```python
from build123d import *

# Parameters (mm, degrees)
SZKIC1_W                                            = 110
SZKIC1_H                                            = 80
DODANIE_WYCI_GNI_CIE1_DEPTH                         = 20
SZKIC4_W                                            = 20
SZKIC4_H                                            = 140
DODANIE_WYCI_GNI_CIE2_DEPTH                         = 75
WYTNIJ_WYCI_GNI_CIE2_DEPTH                          = 56
WYTNIJ_WYCI_GNI_CIE2_DEPTH_BACK                     = 56
POG_BIENIE_WALCOWE_POD_M5_WKR_T_Z_BEM_W_D           = 5.8
POG_BIENIE_WALCOWE_POD_M5_WKR_T_Z_BEM_W_CBORE_D     = 10
POG_BIENIE_WALCOWE_POD_M5_WKR_T_Z_BEM_W_CBORE_DEPTH = 5.4
WYTNIJ_WYCI_GNI_CIE3_DEPTH                          = 111
SZKIC19_R                                           = 2.65
WYTNIJ_WYCI_GNI_CIE4_DEPTH                          = 20
WYTNIJ_WYCI_GNI_CIE5_DEPTH                          = 5
WYTNIJ_WYCI_GNI_CIE6_DEPTH                          = 10


with BuildPart() as part:
    # Szkic1 → Dodanie-wyciągnięcie1 (new body)
    with BuildSketch(Plane.XY):
        Rectangle(SZKIC1_W, SZKIC1_H)
    extrude(amount=DODANIE_WYCI_GNI_CIE1_DEPTH)

    # Szkic4 → Dodanie-wyciągnięcie2 (add)
    with BuildSketch(Plane.XY.offset(20)):
        with Locations((-45, 0)):
            Rectangle(SZKIC4_W, SZKIC4_H)
        with Locations((45, 0)):
            Rectangle(SZKIC4_W, SZKIC4_H)
    extrude(amount=DODANIE_WYCI_GNI_CIE2_DEPTH)

    # Szkic7 → Wytnij-wyciągnięcie2 (cut, two sides)
    with BuildSketch(Plane(origin=(0, 0, 0), x_dir=(0, 0, -1), z_dir=(1, 0, 0))) as wytnij_wyci_gni_cie2_sk:
        Polygon((-95, -70), (-29.716927858, 70), (-95, 70), align=None)
    extrude(amount=WYTNIJ_WYCI_GNI_CIE2_DEPTH, mode=Mode.SUBTRACT)
    extrude(wytnij_wyci_gni_cie2_sk.sketch, amount=-WYTNIJ_WYCI_GNI_CIE2_DEPTH_BACK, mode=Mode.SUBTRACT)

    # Pogłębienie walcowe pod M5 Wkręt z łbem walcowym z gniazdem sześciokątnym2 (through all)
    with Locations(Plane.XY.offset(20)):
        with Locations((-28.25, 11.906323336), (-28.25, -11.906323336), (28.25, -11.906323336), (28.25, 11.906323336)):
            CounterBoreHole(POG_BIENIE_WALCOWE_POD_M5_WKR_T_Z_BEM_W_D / 2, POG_BIENIE_WALCOWE_POD_M5_WKR_T_Z_BEM_W_CBORE_D / 2, POG_BIENIE_WALCOWE_POD_M5_WKR_T_Z_BEM_W_CBORE_DEPTH)

    # Szkic14 → Wytnij-wyciągnięcie3 (cut, through all)
    with BuildSketch(Plane.ZY.offset(55)):
        with BuildLine():
            add(Edge.make_bspline(
                [(38.169293093, 51.873844259), (31.459464211, 48.744999666), (24.920360639, 45.938457736), (20, 40)],
                knots=[0, 0, 0, 0, 1, 1, 1, 1], degree=3))
            Line((38.169293093, 51.873844259), (29.716927858, 70))
            Line((29.716927858, 70), (20, 70))
            Line((20, 70), (20, 40))
        make_face()
        with BuildLine():
            Line((20, -70), (95, -70))
            Line((95, -70), (88.883484502, -56.883090185))
            add(Edge.make_bspline(
                [(88.883484502, -56.883090185), (65.034975945, -68.003832361), (46.153744311, -70.402204642), (20, -40)],
                knots=[0, 0, 0, 0, 1, 1, 1, 1], degree=3))
            Line((20, -40), (20, -70))
        make_face()
    extrude(amount=-WYTNIJ_WYCI_GNI_CIE3_DEPTH, mode=Mode.SUBTRACT)

    # Szkic19 → Wytnij-wyciągnięcie4 (cut)
    with BuildSketch(Plane(origin=(0, 23.884677387, 51.220855951), x_dir=(1, 0, 0), z_dir=(0, 0.422618262, 0.906307787))):
        with Locations((-45, 15.885667625)):
            Circle(SZKIC19_R)
        with Locations((-45, -73.114332375)):
            Circle(SZKIC19_R)
        with Locations((-45, -38.117371303)):
            Circle(SZKIC19_R)
    wytnij_wyci_gni_cie4 = extrude(amount=-WYTNIJ_WYCI_GNI_CIE4_DEPTH, mode=Mode.SUBTRACT)

    # Szkic20 → Wytnij-wyciągnięcie5 (cut)
    with BuildSketch(Plane(origin=(0, 17.545403461, 37.626239145), x_dir=(1, 0, 0), z_dir=(0, 0.422618262, 0.906307787))):
        Polygon((-42.690598923, 19.885667625), (-47.309401077, 19.885667625), (-49.618802154, 15.885667625), (-47.309401077, 11.885667625), (-42.690598923, 11.885667625), (-40.381197846, 15.885667625), align=None)
        Polygon((-42.690598923, -34.117371303), (-47.309401077, -34.117371303), (-49.618802154, -38.117371303), (-47.309401077, -42.117371303), (-42.690598923, -42.117371303), (-40.381197846, -38.117371303), align=None)
        Polygon((-42.690598923, -69.114332375), (-47.309401077, -69.114332375), (-49.618802154, -73.114332375), (-47.309401077, -77.114332375), (-42.690598923, -77.114332375), (-40.381197846, -73.114332375), align=None)
    wytnij_wyci_gni_cie5 = extrude(amount=WYTNIJ_WYCI_GNI_CIE5_DEPTH, mode=Mode.SUBTRACT)

    # Szkic18 → Wytnij-wyciągnięcie6 (cut)
    with BuildSketch(Plane.ZY.offset(55)):
        Polygon((33.753731795, 37.681030189), (37.134677889, 30.430567893), (32.603138954, 28.317476584), (29.22219286, 35.56793888), align=None)
        Polygon((52.044863301, -13.375435824), (55.425809395, -20.625898121), (59.95734833, -18.512806812), (56.576402236, -11.262344516), align=None)
        Polygon((66.835218155, -45.093454166), (70.216164249, -52.343916462), (74.747703184, -50.230825153), (71.36675709, -42.980362857), align=None)
    wytnij_wyci_gni_cie6 = extrude(amount=-WYTNIJ_WYCI_GNI_CIE6_DEPTH, mode=Mode.SUBTRACT)

    # Lustro2: Wytnij-wyciągnięcie4, Wytnij-wyciągnięcie5, Wytnij-wyciągnięcie6 across plane
    add(wytnij_wyci_gni_cie4.mirror(Plane(origin=(0, 0, 0), x_dir=(0, 0, 1), z_dir=(1, 0, 0))), mode=Mode.SUBTRACT)
    add(wytnij_wyci_gni_cie5.mirror(Plane(origin=(0, 0, 0), x_dir=(0, 0, 1), z_dir=(1, 0, 0))), mode=Mode.SUBTRACT)
    add(wytnij_wyci_gni_cie6.mirror(Plane(origin=(0, 0, 0), x_dir=(0, 0, 1), z_dir=(1, 0, 0))), mode=Mode.SUBTRACT)


solid = part.part
```
CAD build for the part. Positions are in the model's coordinates, mm. A direction names the side the tool comes from. Coordinates: 2 decimals unless noted, no trailing zeros. Loops run counter-clockwise (first coordinate to the right, second up) from the corner with the lowest first, then second, coordinate; pieces in that order, holes last. Notation, with made-up numbers: (55, 60.5) - (82, 60.5) arc R33 ccw to (82, 91.5) - close; hole circle Ø3 at (37.25, -16). An arc over 180 degrees is marked (long way). Use CSV: the item, a comma, the result in double quotes. Start each with the question number.
Q1. Cut at B-B, the plane x = 5.5. List the corners of the cut face in (y, z).
Q2. Two-plate mould, pull along X, no slides. Class faces 1 (the flat face through (44.86, -3.266, 63.881)), 2 (the flat face through (41.55, 31.15, 34)), 3 (the cylindrical face through (-31.016, 12.777, 7.198)): +X half, -X half, draft (parallel to the pull), parting line (faces both ways), or undercut.
Q3. Drop flat-ended pins along their axis: P1, Ø21, axis at x = 10, y = -6, coming from the +Z side; P2, Ø22, axis at x = -24, z = 11.5, coming from the +Y side; P3, Ø16, axis at x = 26, z = 13.5, coming from the -Y side. Give the stop position or say it passes through.
Q4. Cut at A-A, the plane x = -28.25. List the corners of the cut face in (y, z).
Q5. 3-axis set-ups, long thin cutter, end or side, ignore diameter. For faces 4 (the flat face through (-1, 40, 10)), 5 (the flat face through (45.04, -19.08, 49.19)), 6 (the flat face through (0, 1, 20)), 7 (the flat face through (-28.3, 8.6, 14.6)): which of +Z, -Z, +X, -X, +Y, -Y reach the whole face in a straight line?
Q6. Probe probe 1 along Y at (x, z) = (28, 18); probe 2 along Y at (x, z) = (28.25, 6); probe 3 along X at (y, z) = (14.5, 11.5). List the from-to ranges inside material, lowest first. Write a range as from..to.
Here are the results:
1,outline,"(-40, 0) - (40, 0) - (40, 20) - (-40, 20) - close"
2,face 1,"draft"
2,face 2,"+X half"
2,face 3,"undercut"
3,P1,"z = 20"
3,P2,"y = 40"
3,P3,"y = -40"
4,outline,"(-40, 0) - (-14.81, 0) - (-14.81, 14.6) - (-16.91, 14.6) - (-16.91, 20) - (-40, 20) - close; (-9.01, 0) - (9.01, 0) - (9.01, 14.6) - (6.91, 14.6) - (6.91, 20) - (-6.91, 20) - (-6.91, 14.6) - (-9.01, 14.6) - close; (14.81, 0) - (40, 0) - (40, 20) - (16.91, 20) - (16.91, 14.6) - (14.81, 14.6) - close"
5,face 4,"-Z, +X, -X, +Y"
5,face 5,"none"
5,face 6,"+Z, +Y, -Y"
5,face 7,"+Z"
6,probe 1,"-40..-16.9, -6.91..6.91, 16.9..40"
6,probe 2,"-40..-14.81, -9.01..9.01, 14.81..40"
6,probe 3,"-55..-29.55, -26.95..26.95, 29.55..55"
